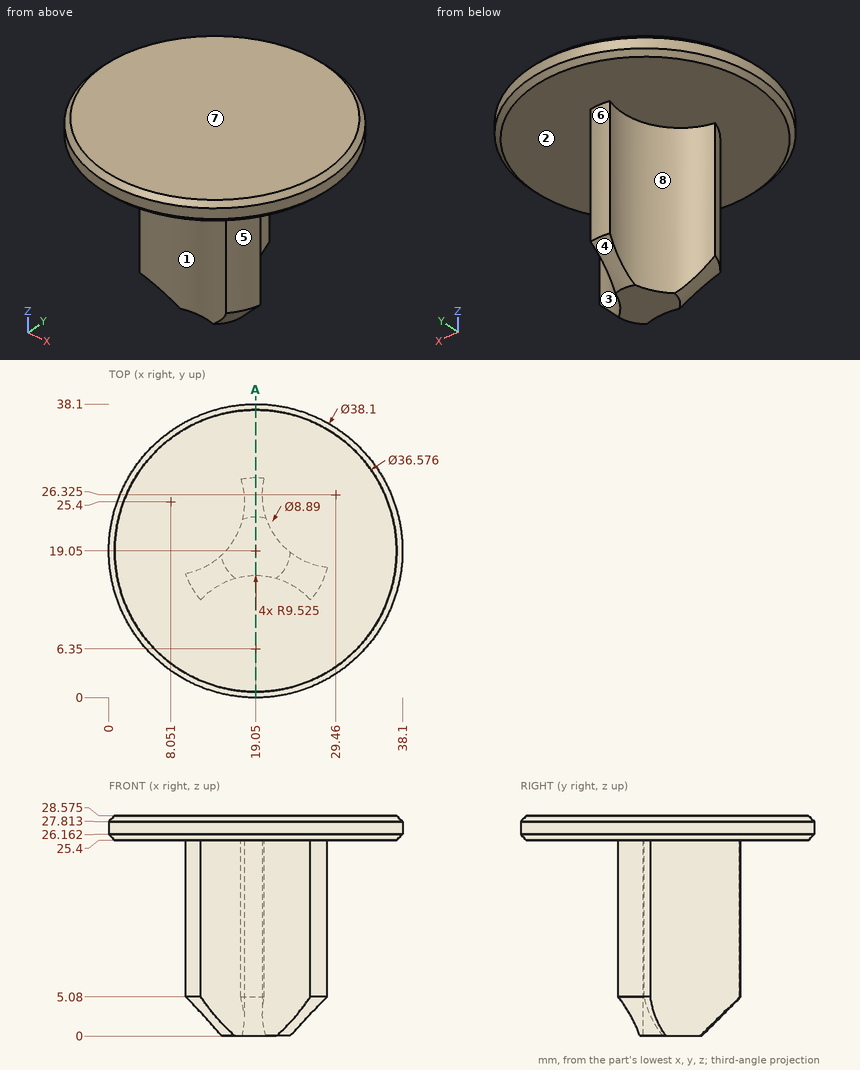
Verification items for this drawing (mm, ordinates from the low corner). A direction names the side the tool comes from. Coordinates: 2 decimals unless noted, no trailing zeros. Loops run counter-clockwise (first coordinate to the right, second up) from the corner with the lowest first, then second, coordinate; pieces in that order, holes last. Notation, with made-up numbers: (12, 76.5) - (51, 76.5) arc R22 ccw to (51, 95.5) - close; hole circle Ø1 at (71.25, 19.25). An arc over 180 degrees is marked (long way). Use one line per item in the form item = value. Start each with the question number.
Item 1: Gauge pin test, flat ends, axial feed: pin 1 (2 mm diameter, centred on y = 15, z = 11, fed in from -X); pin 2 (10 mm diameter, centred on x = 19, z = 16, fed in from -Y) (1 decimal); pin 3 (6 mm diameter, centred on y = 16, z = 11.5, fed in from +X); pin 4 (8 mm diameter, centred on y = 33, z = 10.5, fed in from -X). Record the tip position at first contact, or that the pin passes through.
Item 2: Mould release check, pull along Y, two halves, no side actions. Record for the marked faces 5, 6, 7 and 8: +Y half, -Y half, draft (parallel to the pull), parting line (faces both ways), or undercut.
Item 3: Thickness scan on probe 1 along Z at (x, y) = (34.5, 27) (1 decimal); probe 2 along Y at (x, z) = (19, 13.75) (1 decimal); probe 3 along X at (y, z) = (27, 10.75). Record the ranges inside material, lowest first.
Item 4: Section check A-A, the plane x = 19.05. Enter the section's corners in (y, z) (1 decimal).
Item 5: Tool access check on the marked faces 1, 2, 3 and 4. Record the directions out of +Z, -Z, +X, -X, +Y, -Y that give a thin tool (end or side, any length) a straight path to the whole face; none if there is none.
Computed:
q1.pin_1 = 10.03
q1.pin_2 = 14.4
q1.pin_3 = 28.32
q1.pin_4 = through
q2.face_5 = -Y half
q2.face_6 = +Y half
q2.face_7 = draft
q2.face_8 = undercut
q3.probe_1 = 25.4 to 28.6
q3.probe_2 = 15.9 to 28.6
q3.probe_3 = 17.44 to 19.96
q4.outline = (0, 26.2) - (0.8, 25.4) - (15.9, 25.4) - (15.9, 0) - (23.5, 0) - (28.6, 5.1) - (28.6, 25.4) - (37.3, 25.4) - (38.1, 26.2) - (38.1, 27.8) - (37.3, 28.6) - (0.8, 28.6) - (0, 27.8) - close
q5.face_1 = -Z, -Y
q5.face_2 = -Z
q5.face_3 = -Z, +X
q5.face_4 = -Z, +Y
